```python
from build123d import *

# Parameters (mm, degrees)
ESQUISSE1_R        = 9
ESQUISSE1_R_2      = 2.1
BOSS_EXTRU_1_DEPTH = 4


with BuildPart() as part:
    # Esquisse1 → Boss.-Extru.1 (new body)
    with BuildSketch(Plane.XY):
        with BuildLine():
            Line((14, 0), (14, -18.735720858))
            ThreePointArc((14, -18.735720858), (11.923221563, -23.275360995), (7.13055581, -24.672392215))
            ThreePointArc((7.13055581, -24.672392215), (-11.382149549, -23.123814483), (-29.944297321, -23.875494465))
            ThreePointArc((-29.944297321, -23.875494465), (-37.690469305, -20.031379706), (-37.551840307, -11.384924901))
            ThreePointArc((-37.551840307, -11.384924901), (-22.940340069, 4.071410465), (-3.854513663, 13.458927313))
            ThreePointArc((-3.854513663, 13.458927313), (8.4272418, 11.179516789), (14, 0))
        make_face()
        Circle(ESQUISSE1_R, mode=Mode.SUBTRACT)
        with Locations((6.8, -18.914809013)):
            Circle(ESQUISSE1_R_2, mode=Mode.SUBTRACT)
        with Locations((-30.772589733, -15.817955655)):
            Circle(ESQUISSE1_R_2, mode=Mode.SUBTRACT)
    extrude(amount=BOSS_EXTRU_1_DEPTH)


solid = part.part
```
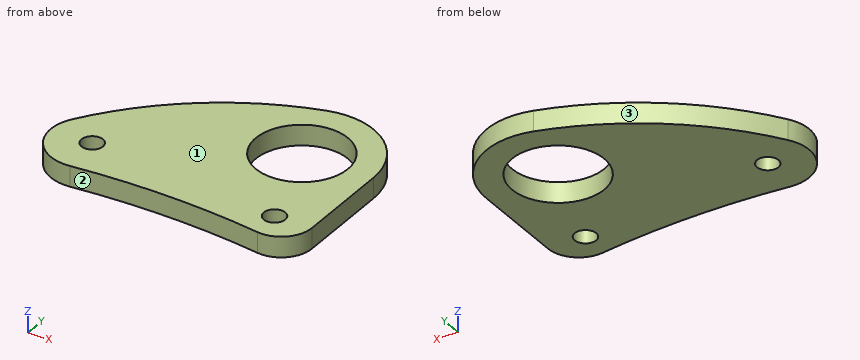
Could you check a few things on this model? Use its own coordinates, in mm. Face numbers are marked on the shaded views. Round coordinates to 2 decimals unless told otherwise and drop trailing zeros. Loops run counter-clockwise (first coordinate to the right, second up) from the corner with the lowest first, then second, coordinate; pieces in that order, holes last. Notation, with made-up numbers: M -35.75,-22.5 L -23.75,-22.5 A15 ccw -23.75,4.5 Z; hole C 19,45 d1. An arc over 180 degrees is marked long. Answer as CSV lines item,"result".
1) Imagine slicing it at B-B on y = -2. List the corners of the cut face in (x, z) for me, and give its area (3 significant figures).
From the geometry:
outline,"M -29.96,0 L -8.77,0 L -8.77,4 L -29.96,4 Z; M 8.77,0 L 14,0 L 14,4 L 8.77,4 Z"
area,"106 mm^2"
2) If I drill on probe 1 along Y at (x, z) = (6.8, 1.25); probe 2 along Y at (x, z) = (-32, 1.5); probe 3 along X at (y, z) = (-2, 0.9), over which ranges is the centre line in solid material (lowest first)?
From the geometry:
probe 1,"-24.62 to -21.01, -16.81 to -5.9, 5.9 to 12.24"
probe 2,"-23.82 to -17.52, -14.11 to -4.16"
probe 3,"-29.96 to -8.77, 8.77 to 14"
3) Imagine slicing it at C-C on x = 6. List the corners of the cut face in (y, z) for me, and give its area (3 significant figures).
From the geometry:
outline,"M -24.51,0 L -20.86,0 L -20.86,4 L -24.51,4 Z; M -16.97,0 L -6.71,0 L -6.71,4 L -16.97,4 Z; M 6.71,0 L 12.65,0 L 12.65,4 L 6.71,4 Z"
area,"79.4 mm^2"
4) We'd pull the mould along X, two halves only. Please class the marked faces 1, 2 and 3: released by +X, released by -X, zero draft, split by the parting line, or undercut.
From the geometry:
face 1,"zero draft"
face 2,"undercut"
face 3,"released by -X"
5) Imagine slicing it at D-D on z = 3.3. List the corners of the cut face in (x, y) for me.
From the geometry:
outline,"M -37.55,-11.38 A8.1 ccw -29.94,-23.88 A150 cw 7.13,-24.67 A6 ccw 14,-18.74 L 14,0 A14 ccw -3.85,13.46 A60 ccw Z; hole C -30.77,-15.82 d4.2; hole C 0,0 d18; hole C 6.8,-18.91 d4.2"
6) Imagine slicing it at A-A on x = -5.5. List the corners of the cut face in (y, z) for me.
From the geometry:
outline,"M -23.37,0 L -7.12,0 L -7.12,4 L -23.37,4 Z; M 7.12,0 L 12.96,0 L 12.96,4 L 7.12,4 Z"
